Geometry: final body of the model. Coordinates: model frame, mm. A direction names the side the tool comes from. Give positions to 0.01 mm unless a question says otherwise; leave off trailing zeros. Write each loop counter-clockwise with the first axis right and the second up, starting at its lowest first coordinate (ties: lowest second). Pieces come first, ordered by that corner, then holes. Notation, with made-up numbers: M 11.5,15 L 19.5,15 A18 cw 19.5,27 Z; hole C 3.5,66 d7. An arc over 180 degrees is marked long. Use a Markdown table: item, result. Add a question column.
1) Section D-D on z = -33. Return the cut outline in (x, y), then the cut area to 3 significant figures.
2) Set-up query: faces 1 (the flat face through (49, -28.738, 59)), 2 (the cylindrical face through (69.076, 60.394, -1.527)), 3 (the flat face through (49, 15.814, 1)). Return all of +Z, -Z, +X, -X, +Y, -Y with unobstructed straight access to the full face (end or side cutting, diameter ignored); none if empty.
3) Line query: line 1 (Y direction, x = 50, z = -46.5); line 2 (Y direction, x = 30, z = 28); line 3 (Z direction, x = 57, y = 2). Output: solid intervals per line, ascending.
4) Section C-C on y = 43.5. Return the cut outline in (x, z), then the cut area to 3 significant figures.
5) Section B-B on x = 12.5. Return the cut outline in (y, z), then the cut area to 3 significant figures.
6) Section A-A on x = 50. Return the cut outline in (y, z), then the cut area to 3 significant figures.
7) Pin query (flat end, axial travel): pin 1 (4 mm diameter, centred on x = 60.5, z = -20, fed in from -Y); pin 2 (3 mm diameter, centred on x = 78.5, z = -26, fed in from +Y); pin 3 (4 mm diameter, centred on x = 44, y = 69, fed in from +Z). Return the tip coordinate at first contact, or that it passes through.
8) Draft query along Z for faces 4 (the flat face through (6.18, 8.07, 46.29)), 5 (the flat face through (100, 23, 0)), 6 (the flat face through (49.369, -1.824, 44.226)). Return one class per face: +Z half, -Z half, draft (parallel to the pull), parting line (faces both ways), or undercut.
```python
from build123d import *

# Parameters (mm, degrees)
BOSS_EXTRUDE1_DEPTH = 100
SKETCH2_R           = 7.5
CUT_EXTRUDE1_DEPTH  = 120
CUT_EXTRUDE2_DEPTH  = 100
SKETCH4_R           = 20
BOSS_EXTRUDE2_DEPTH = 60


with BuildPart() as part:
    # Sketch1 → Boss-Extrude1 (new body)
    with BuildSketch(Plane(origin=(0, 0, 0), x_dir=(0, 0, -1), z_dir=(1, 0, 0))):
        Polygon((-51.437881439, -28.738448854), (-39.5, 15.81433121), (39.5, 15.81433121), (39.5, -29.18566879), (54.5, -29.18566879), (54.5, 30.81433121), (-50.480762114, 30.81433121), (-66.437881439, -28.738448854), align=None)
    extrude(amount=BOSS_EXTRUDE1_DEPTH)

    # Sketch2 → Cut-Extrude1 (cut)
    with BuildSketch(Plane(origin=(0, 0, -54.5), x_dir=(-1, 0, 0), z_dir=(0, 0, -1))):
        with Locations((-50, -12.18566879)):
            Circle(SKETCH2_R)
    extrude(amount=-CUT_EXTRUDE1_DEPTH, mode=Mode.SUBTRACT)

    # Sketch3 → Cut-Extrude2 (cut)
    with BuildSketch(Plane(origin=(0, 30.81433121, 0), x_dir=(1, 0, 0), z_dir=(0, 1, 0))):
        Polygon((10, -66.437881439), (0, -13.684030484), (-18.365032474, -13.684030484), (-18.365032474, -72.107787752), align=None)
        Polygon((-18.365032474, 72.107787752), (10, 66.437881439), (0, 13.684030484), (-18.365032474, 13.684030484), align=None)
        Polygon((90, 66.437881439), (100, 13.684030484), (118.365032474, 13.684030484), (118.365032474, 72.107787752), align=None)
        Polygon((118.365032474, -72.107787752), (90, -66.437881439), (100, -13.684030484), (118.365032474, -13.684030484), align=None)
    extrude(amount=-CUT_EXTRUDE2_DEPTH, mode=Mode.SUBTRACT)

    # Sketch4 → Boss-Extrude2 (add)
    with BuildSketch(Plane(origin=(0, 30.81433121, 0), x_dir=(1, 0, 0), z_dir=(0, 1, 0))):
        with Locations((50, -4.480762114)):
            Circle(SKETCH4_R)
    extrude(amount=BOSS_EXTRUDE2_DEPTH)


solid = part.part
```
Found:
| question | item | result |
|---|---|---|
| 1 | outline | M 3.66,15.81 L 96.34,15.81 L 96.34,30.81 L 3.66,30.81 Z |
| 1 | area | 1,390 mm² |
| 2 | face 1 | +Z, +X, -X, -Y |
| 2 | face 2 | +Y |
| 2 | face 3 | +X, -X, -Y |
| 3 | line 1 | -29.19 to -19.69, -4.69 to 30.81 |
| 3 | line 2 | 15.81 to 30.81 |
| 3 | line 3 | -54.5 to -39.5, 43.2 to 58.2 |
| 4 | outline | C 50,4.48 d40 |
| 4 | area | 1,260 mm² |
| 5 | outline | M -29.19,-54.5 L 30.81,-54.5 L 30.81,50.48 L -28.74,66.44 L -28.74,51.44 L 15.81,39.5 L 15.81,-39.5 L -29.19,-39.5 Z |
| 5 | area | 2,950 mm² |
| 6 | outline | M -29.19,-54.5 L -19.69,-54.5 L -19.69,-39.5 L -29.19,-39.5 Z; M -28.74,51.44 L -19.69,49.01 L -19.69,64.01 L -28.74,66.44 Z; M -4.69,-54.5 L 30.81,-54.5 L 30.81,-15.52 L 90.81,-15.52 L 90.81,24.48 L 30.81,24.48 L 30.81,50.48 L -4.69,59.99 L -4.69,44.99 L 15.81,39.5 L 15.81,-39.5 L -4.69,-39.5 Z |
| 6 | area | 4,900 mm² |
| 7 | pin 1 | y = 15.81 |
| 7 | pin 2 | y = 30.81 |
| 7 | pin 3 | z = 24.08 |
| 8 | face 4 | +Z half |
| 8 | face 5 | draft |
| 8 | face 6 | undercut |
